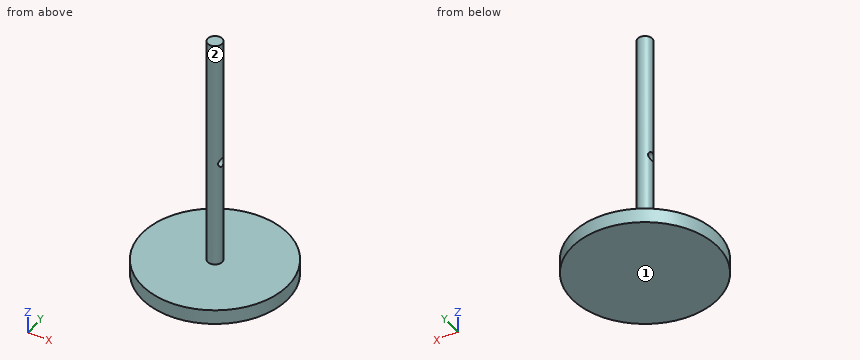
```python
from build123d import *

# Parameters (mm, degrees)
F0_R     = 31.75
F1_DEPTH = 6.35
F2_R     = 3.175
F3_DEPTH = 101.6
F4_R     = 1.905
F5_DEPTH = 12.7


with BuildPart() as f1:
    # F0 (on Top) → F1 (new body)
    with BuildSketch(Plane.XY):
        Circle(F0_R)
    extrude(amount=F1_DEPTH)

    # F2 (on face) → F3 (join)
    with BuildSketch(Plane.XY.offset(6.35)):
        Circle(F2_R)
    extrude(amount=F3_DEPTH)

    # F4 (on Right) → F5 (cut, symmetric)
    with BuildSketch(Plane.YZ):
        with Locations((0, 52.869016)):
            Circle(F4_R)
    extrude(amount=F5_DEPTH, both=True, mode=Mode.SUBTRACT)


solid = f1.part
```
Geometry: final body of the model. Coordinates: model frame, mm. Face numbers are marked on the shaded views. A direction names the side the tool comes from. Coordinates: 2 decimals unless noted, no trailing zeros. Order: outer loops, then holes, each group sorted by start corner. A loop starts at its lowest first (then second) coordinate and runs counter-clockwise, first axis right, second up. Notation, with made-up numbers: (-1.5, -36.75) - (27.5, -36.75) arc R17 ccw to (27.5, -28.75) - close; hole circle Ø11 at (-30, -9.75). An arc over 180 degrees is marked (long way). Return JSON: item names as keys, results as strings. Group by question number.
1. Cut plane D-D (x = -27.5). Output: boundary loops of the cut face in (y, z), plus the area to 3 significant figures.
2. Material intervals for line 1 along Z through (x, y) = (-1, 0); line 2 along Z through (x, y) = (-27.5, 14); line 3 along X through (y, z) = (-2, 26.5), sorted ascending. Write a range as [from, to].
3. Cut plane A-A (y = 0). Output: boundary loops of the cut face in (x, z) (3 decimals), plus the area to 3 significant figures.
4. Cut plane C-C (z = 46.5). Output: boundary loops of the cut face in (x, y) (3 decimals).
5. Pin query (flat end, axial travel): pin 1 (5 mm diameter, centred on y = 0, z = 52.87, fed in from +X) (3 decimals); pin 2 (4 mm diameter, centred on y = 1.5, z = 20, fed in from -X) (3 decimals); pin 3 (3 mm diameter, centred on y = -6.5, z = 57.5, fed in from -X); pin 4 (4 mm diameter, centred on x = -24.5, y = -20, fed in from +Z). Return the tip coordinate at first contact, or that it passes through.
6. Cut plane B-B (x = 0). Output: boundary loops of the cut face in (y, z) (3 decimals).
7. Set-up query: the marked faces 1 and 2. Return all of +Z, -Z, +X, -X, +Y, -Y with unobstructed straight access to the full face (end or side cutting, diameter ignored); none if empty.
Resolved:
{
 "1": {"outline": "(-15.87, 0) - (15.87, 0) - (15.87, 6.35) - (-15.87, 6.35) - close", "area": "202 mm²"},
 "2": {"line 1": "z = [0, 50.96], [54.77, 107.95]", "line 2": "z = [0, 6.35]", "line 3": "x = [-2.47, 2.47]"},
 "3": {"outline": "(-31.75, 0) - (31.75, 0) - (31.75, 6.35) - (3.175, 6.35) - (3.175, 50.964) - (-3.175, 50.964) - (-3.175, 6.35) - (-31.75, 6.35) - close; (-3.175, 54.774) - (3.175, 54.774) - (3.175, 107.95) - (-3.175, 107.95) - close", "area": "1,020 mm²"},
 "4": {"outline": "circle Ø6.35 at (0, 0)"},
 "5": {"pin 1": "stops at x = 3.175", "pin 2": "stops at x = -3.175", "pin 3": "passes through", "pin 4": "stops at z = 6.35"},
 "6": {"outline": "(-31.75, 0) - (31.75, 0) - (31.75, 6.35) - (3.175, 6.35) - (3.175, 107.95) - (-3.175, 107.95) - (-3.175, 6.35) - (-31.75, 6.35) - close; hole circle Ø3.81 at (0, 52.869)"},
 "7": {"face 1": "-Z, +X, -X, +Y, -Y", "face 2": "+Z"}
}
